The listing builds one solid part. Answer for the finished solid, in the listing's coordinates (mm). Face numbers are marked on the shaded views. A direction names the side the tool comes from. Round coordinates to 2 decimals unless told otherwise and drop trailing zeros. Write each loop counter-clockwise with the first axis right and the second up, starting at its lowest first coordinate (ties: lowest second). Pieces come first, ordered by that corner, then holes.
Item 1: Find the intervals of material crossed by probe 1 along X at (y, z) = (-2, 1.5); probe 2 along Y at (x, z) = (-1.75, 2.25); probe 3 along Y at (x, z) = (1.5, 0.25), in increasing order.
Item 2: Find section D-D on x = 2.25. Give the vertices of the cut face in (y, z).
Item 3: Find section A-A on z = 0.25. Give the number of separate pieces and of enclosed holes in the cut face, then the cut area to 3 significant figures.
Item 4: Find section B-B on y = 3. Give the vertices of the cut face in (x, z).
Item 5: For a pull along Y with two mould halves and no side action, classify the marked faces 1, 2, 3 and 4 as +Y half, -Y half, draft (parallel to the pull), parting line (faces both ways), or undercut.
Item 6: A tool of negligible diameter and unlimited length cuts with its end or side. For the marked faces 5, 6 and 7, from which of +Z, -Z, +X, -X, +Y, -Y can it reach the whole face along a straight path? Write none if from no direction.
Item 7: Find section C-C on z = -2.75. Give the vertices of the cut face in (x, y), then the cut area to 3 significant figures.
Item 8: Each of these flat-tipped pins is pushed along its axis until it touches: pin 1 (1.8 mm diameter, centred on x = 6, z = 3, fed in from +Y); pin 2 (1.8 mm diameter, centred on x = 7, z = 1.5, fed in from -Y); pin 3 (1.1 mm diameter, centred on x = -7, z = 2.5, fed in from -Y). Where does it stop, or does it pass through?
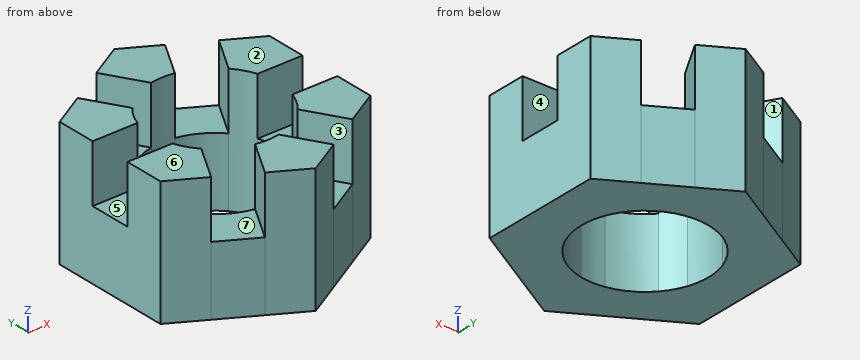
```python
from build123d import *

# Parameters (mm, degrees)
EXTRUDE_1_DEPTH   = 4.5
EXTRUDE_1_2_DEPTH = 4.5
EXTRUDE_1_3_DEPTH = 4.5
EXTRUDE_1_4_DEPTH = 4.5
EXTRUDE_1_5_DEPTH = 4.5
EXTRUDE_1_6_DEPTH = 4.5
EXTRUDE_START     = -5.4
EXTRUDE_2_DEPTH   = 5.4


with BuildPart() as part:
    # Sketch 1 → Extrude 1 (new body)
    with BuildSketch(Plane.XY):
        with BuildLine():
            Line((-8.25, -4.763139721), (-5.553941916, -6.319709581))
            Line((-5.553941916, -6.319709581), (-3.788894246, -3.262557339))
            ThreePointArc((-3.788894246, -3.262557339), (-4.330127019, -2.5), (-4.71990466, -1.65))
            Line((-4.71990466, -1.65), (-8.25, -1.65))
            Line((-8.25, -1.65), (-8.25, -4.763139721))
        make_face()
    extrude(amount=EXTRUDE_1_DEPTH)



with BuildPart() as body_2:
    # Sketch 1 → Extrude 1 2 (new body)
    with BuildSketch(Plane.XY):
        with BuildLine():
            Line((-2.696058084, -7.969709581), (0, -9.526279442))
            Line((0, -9.526279442), (2.696058084, -7.969709581))
            Line((2.696058084, -7.969709581), (0.931010414, -4.912557339))
            ThreePointArc((0.931010414, -4.912557339), (0, -5), (-0.931010414, -4.912557339))
            Line((-0.931010414, -4.912557339), (-2.696058084, -7.969709581))
        make_face()
    extrude(amount=EXTRUDE_1_2_DEPTH)


with BuildPart() as body_3:
    # Sketch 1 → Extrude 1 3 (new body)
    with BuildSketch(Plane.XY):
        with BuildLine():
            Line((3.788894246, -3.262557339), (5.553941916, -6.319709581))
            Line((5.553941916, -6.319709581), (8.25, -4.763139721))
            Line((8.25, -4.763139721), (8.25, -1.65))
            Line((8.25, -1.65), (4.71990466, -1.65))
            ThreePointArc((4.71990466, -1.65), (4.330127019, -2.5), (3.788894246, -3.262557339))
        make_face()
    extrude(amount=EXTRUDE_1_3_DEPTH)


with BuildPart() as body_4:
    # Sketch 1 → Extrude 1 4 (new body)
    with BuildSketch(Plane.XY):
        with BuildLine():
            Line((4.71990466, 1.65), (8.25, 1.65))
            Line((8.25, 1.65), (8.25, 4.763139721))
            Line((8.25, 4.763139721), (5.553941916, 6.319709581))
            Line((5.553941916, 6.319709581), (3.788894246, 3.262557339))
            ThreePointArc((3.788894246, 3.262557339), (4.330127019, 2.5), (4.71990466, 1.65))
        make_face()
    extrude(amount=EXTRUDE_1_4_DEPTH)


with BuildPart() as body_5:
    # Sketch 1 → Extrude 1 5 (new body)
    with BuildSketch(Plane.XY):
        with BuildLine():
            Line((-2.696058084, 7.969709581), (-0.931010414, 4.912557339))
            ThreePointArc((-0.931010414, 4.912557339), (0, 5), (0.931010414, 4.912557339))
            Line((0.931010414, 4.912557339), (2.696058084, 7.969709581))
            Line((2.696058084, 7.969709581), (0, 9.526279442))
            Line((0, 9.526279442), (-2.696058084, 7.969709581))
        make_face()
    extrude(amount=EXTRUDE_1_5_DEPTH)


with BuildPart() as body_6:
    # Sketch 1 → Extrude 1 6 (new body)
    with BuildSketch(Plane.XY):
        with BuildLine():
            Line((-8.25, 4.763139721), (-8.25, 1.65))
            Line((-8.25, 1.65), (-4.71990466, 1.65))
            ThreePointArc((-4.71990466, 1.65), (-4.330127019, 2.5), (-3.788894246, 3.262557339))
            Line((-3.788894246, 3.262557339), (-5.553941916, 6.319709581))
            Line((-5.553941916, 6.319709581), (-8.25, 4.763139721))
        make_face()
    extrude(amount=EXTRUDE_1_6_DEPTH)


with BuildPart() as part_1:
    add(part.part)

    add(body_2.part)  # Extrude 2 merges body 2

    add(body_3.part)  # Extrude 2 merges body 3

    add(body_4.part)  # Extrude 2 merges body 4

    add(body_5.part)  # Extrude 2 merges body 5

    add(body_6.part)  # Extrude 2 merges body 6
    # Sketch 1_4 → Extrude 2 (add)
    with BuildSketch(Plane.XY.offset(EXTRUDE_START)):
        with BuildLine():
            Line((-8.25, 4.763139721), (-8.25, 1.65))
            Line((-8.25, 1.65), (-4.71990466, 1.65))
            ThreePointArc((-4.71990466, 1.65), (-4.330127019, 2.5), (-3.788894246, 3.262557339))
            Line((-3.788894246, 3.262557339), (-5.553941916, 6.319709581))
            Line((-5.553941916, 6.319709581), (-8.25, 4.763139721))
        make_face()
        with BuildLine():
            Line((-5.553941916, 6.319709581), (-3.788894246, 3.262557339))
            ThreePointArc((-3.788894246, 3.262557339), (-2.5, 4.330127019), (-0.931010414, 4.912557339))
            Line((-0.931010414, 4.912557339), (-2.696058084, 7.969709581))
            Line((-2.696058084, 7.969709581), (-5.553941916, 6.319709581))
        make_face()
        with BuildLine():
            Line((-2.696058084, 7.969709581), (-0.931010414, 4.912557339))
            ThreePointArc((-0.931010414, 4.912557339), (0, 5), (0.931010414, 4.912557339))
            Line((0.931010414, 4.912557339), (2.696058084, 7.969709581))
            Line((2.696058084, 7.969709581), (0, 9.526279442))
            Line((0, 9.526279442), (-2.696058084, 7.969709581))
        make_face()
        with BuildLine():
            Line((3.788894246, 3.262557339), (5.553941916, 6.319709581))
            Line((5.553941916, 6.319709581), (2.696058084, 7.969709581))
            Line((2.696058084, 7.969709581), (0.931010414, 4.912557339))
            ThreePointArc((0.931010414, 4.912557339), (2.5, 4.330127019), (3.788894246, 3.262557339))
        make_face()
        with BuildLine():
            Line((4.71990466, 1.65), (8.25, 1.65))
            Line((8.25, 1.65), (8.25, 4.763139721))
            Line((8.25, 4.763139721), (5.553941916, 6.319709581))
            Line((5.553941916, 6.319709581), (3.788894246, 3.262557339))
            ThreePointArc((3.788894246, 3.262557339), (4.330127019, 2.5), (4.71990466, 1.65))
        make_face()
        with BuildLine():
            Line((4.71990466, -1.65), (8.25, -1.65))
            Line((8.25, -1.65), (8.25, 1.65))
            Line((8.25, 1.65), (4.71990466, 1.65))
            ThreePointArc((4.71990466, 1.65), (4.929478842, 0.836802456), (5, 0))
            ThreePointArc((5, 0), (4.929478842, -0.836802456), (4.71990466, -1.65))
        make_face()
        with BuildLine():
            Line((3.788894246, -3.262557339), (5.553941916, -6.319709581))
            Line((5.553941916, -6.319709581), (8.25, -4.763139721))
            Line((8.25, -4.763139721), (8.25, -1.65))
            Line((8.25, -1.65), (4.71990466, -1.65))
            ThreePointArc((4.71990466, -1.65), (4.330127019, -2.5), (3.788894246, -3.262557339))
        make_face()
        with BuildLine():
            Line((0.931010414, -4.912557339), (2.696058084, -7.969709581))
            Line((2.696058084, -7.969709581), (5.553941916, -6.319709581))
            Line((5.553941916, -6.319709581), (3.788894246, -3.262557339))
            ThreePointArc((3.788894246, -3.262557339), (2.5, -4.330127019), (0.931010414, -4.912557339))
        make_face()
        with BuildLine():
            Line((-2.696058084, -7.969709581), (0, -9.526279442))
            Line((0, -9.526279442), (2.696058084, -7.969709581))
            Line((2.696058084, -7.969709581), (0.931010414, -4.912557339))
            ThreePointArc((0.931010414, -4.912557339), (0, -5), (-0.931010414, -4.912557339))
            Line((-0.931010414, -4.912557339), (-2.696058084, -7.969709581))
        make_face()
        with BuildLine():
            Line((-5.553941916, -6.319709581), (-2.696058084, -7.969709581))
            Line((-2.696058084, -7.969709581), (-0.931010414, -4.912557339))
            ThreePointArc((-0.931010414, -4.912557339), (-2.5, -4.330127019), (-3.788894246, -3.262557339))
            Line((-3.788894246, -3.262557339), (-5.553941916, -6.319709581))
        make_face()
        with BuildLine():
            Line((-8.25, -4.763139721), (-5.553941916, -6.319709581))
            Line((-5.553941916, -6.319709581), (-3.788894246, -3.262557339))
            ThreePointArc((-3.788894246, -3.262557339), (-4.330127019, -2.5), (-4.71990466, -1.65))
            Line((-4.71990466, -1.65), (-8.25, -1.65))
            Line((-8.25, -1.65), (-8.25, -4.763139721))
        make_face()
        with BuildLine():
            Line((-8.25, 1.65), (-8.25, -1.65))
            Line((-8.25, -1.65), (-4.71990466, -1.65))
            ThreePointArc((-4.71990466, -1.65), (-5, 0), (-4.71990466, 1.65))
            Line((-4.71990466, 1.65), (-8.25, 1.65))
        make_face()
    extrude(amount=EXTRUDE_2_DEPTH)


solid = part_1.part
```
Check values:
1. probe 1: x = -8.25 to -4.58, 4.58 to 8.25
1. probe 2: y = -8.52 to -6.33, 6.33 to 8.52
1. probe 3: y = -8.66 to -5.9, 5.9 to 8.66
2. outline: (-8.23, -5.4) - (-4.47, -5.4) - (-4.47, 0) - (-7.2, 0) - (-7.2, 4.5) - (-8.23, 4.5) - close; (4.47, -5.4) - (8.23, -5.4) - (8.23, 4.5) - (7.2, 4.5) - (7.2, 0) - (4.47, 0) - close
3. separate pieces: 6
3. enclosed holes: 0
3. area: 91.1 mm2
4. outline: (-8.25, -5.4) - (-4, -5.4) - (-4, 4.5) - (-8.25, 4.5) - close; (4, -5.4) - (8.25, -5.4) - (8.25, 4.5) - (4, 4.5) - close
5. face 1: +Y half
5. face 2: draft
5. face 3: -Y half
5. face 4: undercut
6. face 5: +Z, +X, -X
6. face 6: +Z, +X, -X, +Y, -Y
6. face 7: +Z
7. outline: (-8.25, -4.76) - (0, -9.53) - (8.25, -4.76) - (8.25, 4.76) - (0, 9.53) - (-8.25, 4.76) - close; hole circle Ø10 at (0, 0)
7. area: 157 mm2
8. pin 1: stops at y = 6.32
8. pin 2: stops at y = -6
8. pin 3: stops at y = -5.8
